Source: CAD feature listing. Evaluate the final solid. Frame: model axes, mm. Face numbers are marked on the shaded views. Coordinates: 2 decimals unless noted, no trailing zeros. Write each loop counter-clockwise with the first axis right and the second up, starting at its lowest first coordinate (ties: lowest second). Pieces come first, ordered by that corner, then holes. Notation, with made-up numbers: M -17,47 L -3,47 A31 ccw -3,75 Z; hole C -3.75,55.25 d8. An arc over 180 degrees is marked long. Answer as CSV lines item,"result". Start each with the question number.
1. Section C-C on z = 78.5. Return the cut outline in (x, y).
2. Mould query, pull axis Z, two halves, no side actions, for the marked faces 1 and 2. Classes: pulls with the +Z half, pulls with the -Z half, needs draft (parallel to the pull), parting line crosses it, or undercut.
3. Line query: probe 1 along Y at (x, z) = (3.75, 100.75); probe 2 along Z at (x, y) = (4.5, -2.75); probe 3 along Z at (x, y) = (4.5, -1). Output: solid intervals per line, ascending. Write a range as [from, to].
4. Contact query for flat-ended pins moving along their axis: pin 1 Ø1.5 at (x, y) = (1, 6.5) entering from -Z; pin 2 Ø5 at (y, z) = (-6.5, 69.5) entering from +X; pin 3 Ø6 at (x, y) = (3, -10) entering from -Z; pin 4 Ø8 at (y, z) = (0, 100.75) entering from +X. Output: stop coordinate, or through.
5. Section B-B on x = 5.25. Return the cut outline in (y, z), plus the area to 3 significant figures.
6. Section A-A on y = 0. Return the cut outline in (x, z).
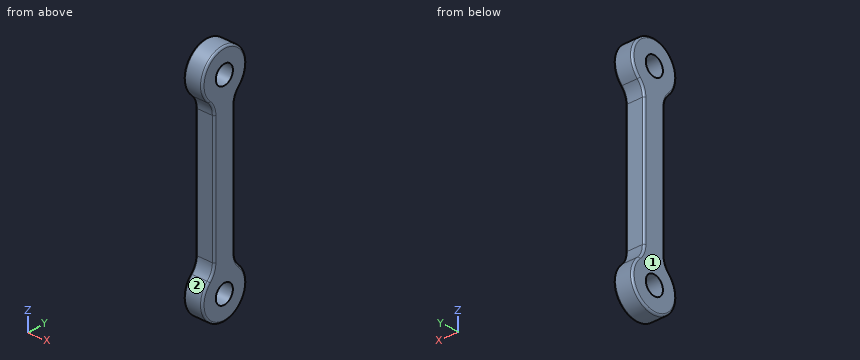
```python
from build123d import *

# Parameters (mm, degrees)
SKETCH_1_R      = 5.05
EXTRUDE_1_DEPTH = 10
FILLET_1_R      = 1


with BuildPart() as part:
    # 草图1 → 凸台-拉伸1 (new body)
    with BuildSketch(Plane(origin=(0, 0, 0), x_dir=(0, 0, -1), z_dir=(1, 0, 0))):
        with BuildLine():
            Line((-84.227288358, 6), (-16.522711642, 6))
            ThreePointArc((-16.522711642, 6), (-12.621764154, 6.792252789), (-9.338923971, 9.043478261))
            ThreePointArc((-9.338923971, 9.043478261), (13, 0), (-9.338923971, -9.043478261))
            ThreePointArc((-9.338923971, -9.043478261), (-12.621764154, -6.792252789), (-16.522711642, -6))
            Line((-16.522711642, -6), (-84.227288358, -6))
            ThreePointArc((-84.227288358, -6), (-88.128235846, -6.792252789), (-91.411076029, -9.043478261))
            ThreePointArc((-91.411076029, -9.043478261), (-113.75, 0), (-91.411076029, 9.043478261))
            ThreePointArc((-91.411076029, 9.043478261), (-88.128235846, 6.792252789), (-84.227288358, 6))
        make_face()
        with Locations((-100.75, 0)):
            Circle(SKETCH_1_R, mode=Mode.SUBTRACT)
        Circle(SKETCH_1_R, mode=Mode.SUBTRACT)
    extrude(amount=EXTRUDE_1_DEPTH)

    # 圆角1
    fillet_1_edges = [part.edges().sort_by_distance(p)[0] for p in [
        (0, 6, 50.375),
        (0, 6.792252789, 12.621764154),
        (0, 0, -13),
        (0, -6.792252789, 12.621764154),
        (10, 6.792252789, 12.621764154),
        (10, 6, 50.375),
        (10, 6.792252789, 88.128235846),
        (10, 0, 113.75),
        (10, -6.792252789, 88.128235846),
        (10, -6, 50.375),
        (10, -6.792252789, 12.621764154),
        (0, -6, 50.375),
        (10, 0, -13),
        (0, -6.792252789, 88.128235846),
        (0, 0, 113.75),
        (0, 6.792252789, 88.128235846),
    ]]
    fillet(fillet_1_edges, radius=FILLET_1_R)


solid = part.part
```
Values:
1,outline,"M 0,-5 A1 ccw 1,-6 L 9,-6 A1 ccw 10,-5 L 10,5 A1 ccw 9,6 L 1,6 A1 ccw 0,5 Z"
2,face 1,"needs draft"
2,face 2,"undercut"
3,probe 1,"[-13, -5.05], [5.05, 13]"
3,probe 2,"[-12.71, -4.24], [4.24, 96.51], [104.99, 113.46]"
3,probe 3,"[-12.96, -4.95], [4.95, 95.8], [105.7, 113.71]"
4,pin 1,"z = -11.66"
4,pin 2,"x = 10"
4,pin 3,"z = -10.95"
4,pin 4,"through"
5,outline,"M -9.04,9.34 A13 ccw long 9.04,9.34 A10 cw 6,16.52 L 6,84.23 A10 cw 9.04,91.41 A13 ccw long -9.04,91.41 A10 cw -6,84.23 L -6,16.52 A10 cw Z; hole C 0,0 d10.1; hole C 0,100.75 d10.1"
5,area,"1,820 mm²"
6,outline,"M 0,-12 A1 ccw 1,-13 L 9,-13 A1 ccw 10,-12 L 10,-5.05 L 0,-5.05 Z; M 0,5.05 L 10,5.05 L 10,95.7 L 0,95.7 Z; M 0,105.8 L 10,105.8 L 10,112.75 A1 ccw 9,113.75 L 1,113.75 A1 ccw 0,112.75 Z"
